Read the model definition and answer for the solid it produces. Units are mm, in the model's axes. Face numbers are marked on the shaded views. A direction names the side the tool comes from. Round coordinates to 2 decimals unless told otherwise and drop trailing zeros. Write each loop counter-clockwise with the first axis right and the second up, starting at its lowest first coordinate (ties: lowest second). Pieces come first, ordered by that corner, then holes. Notation, with made-up numbers: (-35, 72) - (-18, 72) arc R12 cw to (-18, 93) - close; hole circle Ø10 at (-31.75, 61.25). An arc over 180 degrees is marked (long way). One line per item, written item: value. Start each with the question number.
(1) A cutting plane is placed at B-B, the plane x = -6. Determine the outline of the cut face in (y, z) (3 decimals).
(2) A cutting plane is placed at C-C, the plane y = -1. State how many separate pieces and enclosed holes the cut face has, plus the area to 3 significant figures.
(3) The mould has two halves that part along Z. Classify the marked faces 1, 2 and 3: +Z half, -Z half, draft (parallel to the pull), parting line (faces both ways), or undercut.
(4) For the marked faces 4 and 5, determine the directions among +Z, -Z, +X, -X, +Y, -Y from which every point of the face is accessible in a straight line to the end or side of a thin tool.
(5) A flat-ended cylindrical pin translates along its axis: pin 1 Ø5 at (x, z) = (-5, 10.5) entering from -Y. Find the tip coordinate at first contact, or state that the pin passes through.
(6) Find the intervals of material crossed by L1, parallel to X at y = -1, z = 6 (3 decimals); L2, parallel to X at y = -1, z = 2.75 (3 decimals); L3, parallel to Y at x = 6, z = 4.5 (3 decimals), in increasing order.
(7) A cutting plane is placed at A-A, the plane x = 1. Determine the outline of the cut face in (y, z).
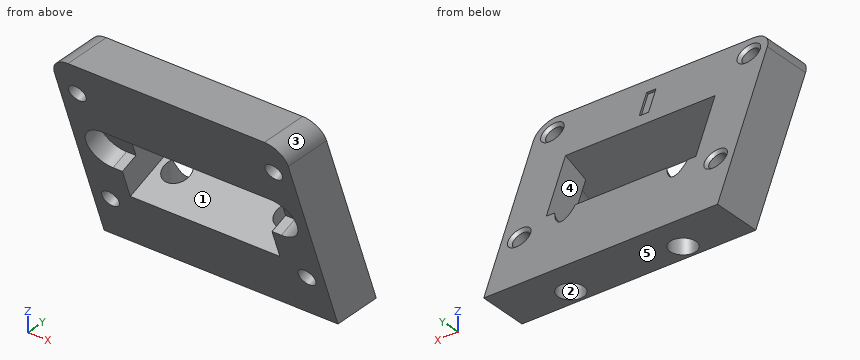
Autodesk Inventor part; units mm, degrees
ref_plane "YZ Plane" through (0, 0, 0) normal (1, 0, 0) x (0, 1, 0)
ref_plane "XZ Plane" through (0, 0, 0) normal (0, 1, 0) x (-1, 0, 0)
ref_plane "XY Plane" through (0, 0, 0) normal (0, 0, 1) x (1, 0, 0)
sketch "Skizze1" plane through (0, 0, 0) normal (1, 0, 0) x (0, 1, 0)
  line L0 (2.6604, 0) -> (-2.6604, 0)
  line L1 (-2.6604, 0) -> (-10.3038, 21)
  line L2 (-10.3038, 21) -> (-4.9829, 21)
  line L3 (-4.9829, 21) -> (2.6604, 0)
  point P0 (0, 0)
  point P1 (0, 0)
  dimension "d1" = 21
  dimension "d2" = 70
  dimension "d33" = 5
extrude "Extrusion1" add sketch "Skizze1" along normal mid plane 25
sketch "Skizze3" plane through (-12.5, -2.6604, 0) normal (0, -0.9396926, -0.3420201) x (1, 0, 0)
  line L0 (25, 0) -> (0, 0)
  line L1 (25, 22.3477) -> (25, 0)
  line L2 (25, 22.3477) -> (0, 22.3477)
  line L3 (0, 0) -> (0, 22.3477)
  line L4 (3.5, 12) -> (21.5, 12) construction
  line L5 (3.5, 9.7) -> (21.5, 9.7)
  line L6 (21.5, 14.3) -> (3.5, 14.3)
  arc A0 (3.5, 14.3) -> (3.5, 9.7) centre (3.5, 12) ccw
  arc A1 (21.5, 9.7) -> (21.5, 14.3) centre (21.5, 12) ccw
  line L7 (12.5, 22.3477) -> (12.5, 0) construction
  point P0 (12.5, -0.9099)
  point P1 (12.5, 12)
  dimension "d10" = 4.6
  dimension "d11" = 18
  dimension "d12" = 12
extrude "Extrusion3" cut sketch "Skizze3" against normal blind 2 contours A0 L6 A1 L5
sketch "Skizze4" plane through (-12.5, -2.6604, 0) normal (0, -0.9396926, -0.3420201) x (1, 0, 0)
  line L0 (2, 18.5) -> (23, 18.5) construction
  line L1 (23, 18.5) -> (23, 5) construction
  line L2 (23, 5) -> (2, 5) construction
  line L3 (2, 5) -> (2, 18.5) construction
  line L4 (3.5, 14.3) -> (21.5, 14.3)
  arc A0 (21.5, 9.7) -> (21.5, 14.3) centre (21.5, 12) ccw
  line L5 (21.5, 9.7) -> (3.5, 9.7)
  arc A1 (3.5, 14.3) -> (3.5, 9.7) centre (3.5, 12) ccw
  line L6 (25, 0) -> (0, 0)
  line L7 (25, 22.3477) -> (25, 0)
  line L8 (25, 22.3477) -> (0, 22.3477)
  line L9 (0, 0) -> (0, 22.3477)
  line L10 (25, 22.3477) -> (0, 22.3477) construction
  line L11 (12.5, 22.3477) -> (12.5, 0) construction
  line L12 (25, 0) -> (0, 0) construction
  point P0 (12.5, -0.9099)
  dimension "d15" = 21
  dimension "d16" = 13.5
  dimension "d34" = 7
hole "Bohrung1" at (-10.5, -8.9878, 17.3843) at (10.5, -8.9878, 17.3843) at (10.5, -4.3705, 4.6985) at (-10.5, -4.3705, 4.6985) direction (0, 0.9396926, 0.3420201) diameter 1.85 end through all
sketch "Skizze5" plane through (12.5, 2.6604, 0) normal (0, 0, -1) x (-1, 0, 0)
  line L0 (25, 0) -> (0, 0)
  line L1 (0, -5.3209) -> (0, 0)
  line L2 (0, -5.3209) -> (25, -5.3209)
  line L3 (25, 0) -> (25, -5.3209)
  line L4 (0, -5.3209) -> (0, 0) construction
  line L5 (25, 0) -> (25, -5.3209) construction
  line L6 (0, -3.6604) -> (25, -3.6604) construction
  line L7 (25, 0) -> (0, 0) construction
  line L8 (12.5, 0) -> (12.5, -5.3209) construction
  point P0 (12.5, -2.6604)
  point P1 (6.5, -3.6604)
  point P2 (18.5, -3.6604)
  dimension "d25" = 12
  dimension "d43" = 1
hole "Bohrung2" at (6, -1, 0) at (-6, -1, 0) direction (0, 0, 1) diameter 2.75 end through all
sketch "Skizze6" plane through (-12.5, -2.6604, 0) normal (0, -0.9396926, -0.3420201) x (1, 0, 0)
  line L0 (21.5, 9.7) -> (3.5, 9.7)
  arc A0 (21.5, 9.7) -> (21.5, 14.3) centre (21.5, 12) ccw
  line L1 (3.5, 14.3) -> (21.5, 14.3)
  arc A1 (3.5, 14.3) -> (3.5, 9.7) centre (3.5, 12) ccw
  line L2 (3.5, 14.3) -> (21.5, 14.3)
  line L3 (4.5, 14.3) -> (20.5, 14.3)
  line L4 (20.5, 14.3) -> (20.5, 6.5)
  line L5 (20.5, 6.5) -> (4.5, 6.5)
  line L6 (4.5, 6.5) -> (4.5, 14.3)
  line L7 (21.5, 9.7) -> (3.5, 9.7) construction
  line L8 (12.5, 9.7) -> (12.5, 14.3) construction
  point P0 (12.5, -0.9099)
  dimension "d35" = 16
  dimension "d36" = 7.8
extrude "Extrusion4" cut sketch "Skizze6" against normal through all contours L4 L5 L6 L0 | L0 L6 L1 L4
fillet "Rundung1" radius 2 2 edges at (-12.5, -7.6434, 21) (12.5, -7.6434, 21)
chamfer "Fase1" distance 0.3 angle 45 4 edges at (10.5, 0.0115, 7.2778) (10.5, -4.6057, 19.9636) (-10.5, -4.6057, 19.9636) (-10.5, 0.0115, 7.2778)
sketch "Skizze7" plane through (-12.5, 2.6604, 0) normal (0, 0.9396926, 0.3420201) x (1, 0, 0)
  circle A0 centre (2, -20.3199) radius 1.225
  circle A1 centre (23, -6.8199) radius 1.225
  ellipse E0 centre (23, -20.2194) end of major axis (23, -22.3477) minor radius 2 (23, -22.3477) -> (25, -20.2194) ccw
  line L0 (25, 0) -> (25, -20.2194)
  line L1 (0, 0) -> (25, 0)
  line L2 (0, -20.2194) -> (0, 0)
  ellipse E1 centre (2, -20.2194) end of major axis (2, -22.3477) minor radius 2 (0, -20.2194) -> (2, -22.3477) ccw
  line L3 (23, -22.3477) -> (2, -22.3477)
  line L4 (19.6075, -8.3199) -> (20.5, -8.3199)
  line L5 (20.5, -8.3199) -> (20.5, -16.1199)
  line L6 (20.5, -16.1199) -> (4.5, -16.1199)
  line L7 (4.5, -16.1199) -> (4.5, -8.3199)
  line L8 (4.5, -8.3199) -> (5.3925, -8.3199)
  ellipse E2 centre (6.5, -10.7024) end of major axis (6.5, -6.6822) minor radius 1.375 (7.6075, -8.3199) -> (5.3925, -8.3199) ccw
  line L9 (7.6075, -8.3199) -> (17.3925, -8.3199)
  ellipse E3 centre (18.5, -10.7024) end of major axis (18.5, -6.6822) minor radius 1.375 (19.6075, -8.3199) -> (17.3925, -8.3199) ccw
  circle A2 centre (23, -20.3199) radius 1.225
  circle A3 centre (2, -6.8199) radius 1.225
  line L10 (13, -17.5949) -> (12, -17.5949)
  line L11 (12, -17.5949) -> (12, -20.5949)
  line L12 (12, -20.5949) -> (13, -20.5949)
  line L13 (13, -20.5949) -> (13, -17.5949)
  line L14 (13, -17.5949) -> (12, -20.5949) construction
  line L15 (12, -17.5949) -> (13, -20.5949) construction
  point P0 (12.5, -0.9099)
  point P1 (12.5, -19.0949)
  dimension "d44" = 1
  dimension "d45" = 3
extrude "Extrusion5" cut sketch "Skizze7" against normal blind 0.2 contours L13 L12 L11 L10
properties part number "Kamerahalter Vorne geneigt"
Here are the results:
1. outline: (-10.304, 21) - (-7.551, 13.438) - (-2.853, 15.148) - (-4.983, 21) - close; (-4.884, 6.108) - (-2.66, 0) - (-2.375, 0) - (-2.375, 7.021) - close; (0.375, 0) - (2.66, 0) - (0.375, 6.279) - close
2. separate pieces: 3
2. enclosed holes: 2
2. area: 164 mm²
3. face 1: undercut
3. face 2: draft
3. face 3: +Z half
4. face 4: none
4. face 5: -Z, +X, -X, +Y, -Y
5. pin 1: through
6. L1: -12.5 to -11.422, -9.578 to -7.375, -4.625 to 4.625, 7.375 to 9.578, 11.422 to 12.5
6. L2: -12.5 to -7.375, -4.625 to 4.625, 7.375 to 12.5
6. L3: -4.298 to -2.375, 0.375 to 1.023
7. outline: (-10.3, 21) - (-7.55, 13.44) - (-2.85, 15.15) - (-4.98, 21) - close; (-4.88, 6.11) - (-2.66, 0) - (2.66, 0) - (-0.19, 7.82) - close
